from build123d import *

# Parameters (mm, degrees)
SKETCH1_W                = 82.55
SKETCH1_H                = 43.434
BOSS_EXTRUDE1_DEPTH      = 5.334
CUT_EXTRUDE1_START       = -88.085249325
CUT_EXTRUDE1_OUTLINE_W   = 5.334
CUT_EXTRUDE1_OUTLINE_H   = 5.334
CUT_EXTRUDE1_DEPTH       = 16.51
CUT_EXTRUDE1_START_2     = -55.065249325
CUT_EXTRUDE1_2_OUTLINE_W = 5.334
CUT_EXTRUDE1_2_OUTLINE_H = 5.334
CUT_EXTRUDE1_2_DEPTH     = 16.51
CUT_EXTRUDE1_START_3     = -22.045249325
CUT_EXTRUDE1_3_OUTLINE_W = 5.334
CUT_EXTRUDE1_3_OUTLINE_H = 5.334
CUT_EXTRUDE1_3_DEPTH     = 16.51
SKETCH3_W                = 5.334
SKETCH3_H                = 9.525
CUT_EXTRUDE2_DEPTH       = 93.990910348
SKETCH4_R                = 3.81
CUT_EXTRUDE3_DEPTH       = 93.990910348
SKETCH5_W                = 16.51
SKETCH5_H                = 5.334
BOSS_EXTRUDE2_DEPTH      = 9.144
SKETCH6_W                = 7.700463705
SKETCH6_H                = 5.334
SKETCH6_W_2              = 7.700463706
CUT_EXTRUDE4_DEPTH       = 93.990910348


# Read off the part's stored shape, not the designer's step: Cut-Extrude1
with BuildPart() as part:
    # Sketch1 → Boss-Extrude1 (new body)
    with BuildSketch(Plane.XY):
        with Locations((-46.810249325, -7.606142782)):
            Rectangle(SKETCH1_W, SKETCH1_H)
    extrude(amount=BOSS_EXTRUDE1_DEPTH)

    # Cut-Extrude1 outline → Cut-Extrude1 (cut)
    with BuildSketch(Plane.YZ.offset(CUT_EXTRUDE1_START)):
        with Locations((11.443857218, 2.667)):
            Rectangle(CUT_EXTRUDE1_OUTLINE_W, CUT_EXTRUDE1_OUTLINE_H)
    extrude(amount=CUT_EXTRUDE1_DEPTH, mode=Mode.SUBTRACT)

    # Cut-Extrude1 2 outline → Cut-Extrude1 2 (cut)
    with BuildSketch(Plane.YZ.offset(CUT_EXTRUDE1_START_2)):
        with Locations((11.443857218, 2.667)):
            Rectangle(CUT_EXTRUDE1_2_OUTLINE_W, CUT_EXTRUDE1_2_OUTLINE_H)
    extrude(amount=CUT_EXTRUDE1_2_DEPTH, mode=Mode.SUBTRACT)

    # Cut-Extrude1 3 outline → Cut-Extrude1 3 (cut)
    with BuildSketch(Plane.YZ.offset(CUT_EXTRUDE1_START_3)):
        with Locations((11.443857218, 2.667)):
            Rectangle(CUT_EXTRUDE1_3_OUTLINE_W, CUT_EXTRUDE1_3_OUTLINE_H)
    extrude(amount=CUT_EXTRUDE1_3_DEPTH, mode=Mode.SUBTRACT)

    # Sketch3 → Cut-Extrude2 (cut, through all)
    with BuildSketch(Plane.XY.offset(5.334)):
        with Locations((-79.166667411, -24.560642782)):
            Rectangle(SKETCH3_W, SKETCH3_H)
        with Locations((-79.166667411, -5.510642782)):
            Rectangle(SKETCH3_W, SKETCH3_H)
        with Locations((-14.453831238, -5.510642782)):
            Rectangle(SKETCH3_W, SKETCH3_H)
        with Locations((-14.453831238, -24.560642782)):
            Rectangle(SKETCH3_W, SKETCH3_H)
    extrude(amount=-CUT_EXTRUDE2_DEPTH, mode=Mode.SUBTRACT)

    # Sketch4 → Cut-Extrude3 (cut, through all)
    with BuildSketch(Plane.XY.offset(5.334)):
        with Locations((-46.810249325, -6.463142782)):
            Circle(SKETCH4_R)
    extrude(amount=-CUT_EXTRUDE3_DEPTH, mode=Mode.SUBTRACT)

    # Sketch5 → Boss-Extrude2 (add)
    with BuildSketch(Plane(origin=(0, 14.110857218, 0), x_dir=(1, 0, 0), z_dir=(0, 1, 0))):
        with Locations((-63.320249325, -2.667)):
            Rectangle(SKETCH5_W, SKETCH5_H)
        with Locations((-30.300249325, -2.667)):
            Rectangle(SKETCH5_W, SKETCH5_H)
    extrude(amount=BOSS_EXTRUDE2_DEPTH)

    # Sketch6 → Cut-Extrude4 (cut, through all)
    with BuildSketch(Plane.XY.offset(5.334)):
        with Locations((-63.360481178, 16.777857218)):
            Rectangle(SKETCH6_W, SKETCH6_H)
        with Locations((-30.260017472, 16.777857218)):
            Rectangle(SKETCH6_W_2, SKETCH6_H)
    extrude(amount=-CUT_EXTRUDE4_DEPTH, mode=Mode.SUBTRACT)


solid = part.part
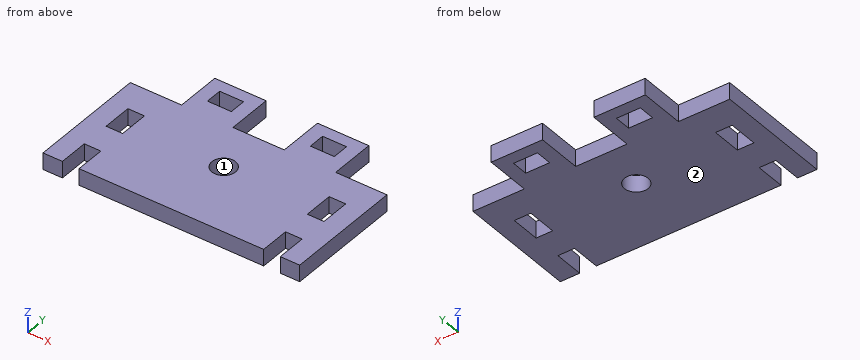
Part model, mm, in its own coordinate system. Face numbers are marked on the shaded views. Coordinates: 2 decimals unless noted, no trailing zeros. Order: outer loops, then holes, each group sorted by start corner. A loop starts at its lowest first (then second) coordinate and runs counter-clockwise, first axis right, second up.
(1) Slice it at B-B, the plane x = -30. Write the cut outline in (y, z), and give its area (3 significant figures).
Check sheet entries:
outline: (-29.32, 0) - (14.11, 0) - (14.11, 5.33) - (-29.32, 5.33) - close; (19.44, 0) - (23.25, 0) - (23.25, 5.33) - (19.44, 5.33) - close
area: 252 mm2
(2) Pull direction X, two halves, no side cores. Call the marked faces 1 and 2: pulls with the +X half, pulls with the -X half, needs draft (parallel to the pull), parting line crosses it, or undercut.
Check sheet entries:
face 1: undercut
face 2: needs draft
(3) Slice it at C-C, the plane y = 16. Write the cut outline in (x, z), and give its area (3 significant figures).
Check sheet entries:
outline: (-71.58, 0) - (-67.21, 0) - (-67.21, 5.33) - (-71.58, 5.33) - close; (-59.51, 0) - (-55.07, 0) - (-55.07, 5.33) - (-59.51, 5.33) - close; (-38.56, 0) - (-34.11, 0) - (-34.11, 5.33) - (-38.56, 5.33) - close; (-26.41, 0) - (-22.05, 0) - (-22.05, 5.33) - (-26.41, 5.33) - close
area: 94.0 mm2
(4) Slice it at A-A, the plane y = -25. Write the cut outline in (x, z).
Check sheet entries:
outline: (-88.09, 0) - (-81.83, 0) - (-81.83, 5.33) - (-88.09, 5.33) - close; (-76.5, 0) - (-17.12, 0) - (-17.12, 5.33) - (-76.5, 5.33) - close; (-11.79, 0) - (-5.54, 0) - (-5.54, 5.33) - (-11.79, 5.33) - close
(5) Pin check, flat tips, straight feed: pin 1 Ø1.6 at (y, z) = (17, 4) entering from -X; pin 2 Ø2.5 at (x, z) = (-76.5, 3) entering from +Y; pin 3 Ø1.6 at (y, z) = (16.5, 3.5) entering from +X. Stop position of each tip, or through.
Check sheet entries:
pin 1: stops at x = -71.58
pin 2: stops at y = 8.78
pin 3: stops at x = -22.05
(6) Probe L1, parallel to X at y = -22, z = 2.25; L2, parallel to X at y = -6.5, z = 1; L3, parallel to Y at x = -28.5, z = 1.55. List the from-to ranges inside material, lowest first.
Check sheet entries:
L1: x = -88.09 to -81.83, -76.5 to -17.12, -11.79 to -5.54
L2: x = -88.09 to -81.83, -76.5 to -50.62, -43 to -17.12, -11.79 to -5.54
L3: y = -29.32 to 14.11, 19.44 to 23.25
(7) Slice it at D-D, the plane x = -20. Write the cut outline in (y, z).
Check sheet entries:
outline: (-29.32, 0) - (8.78, 0) - (8.78, 5.33) - (-29.32, 5.33) - close
